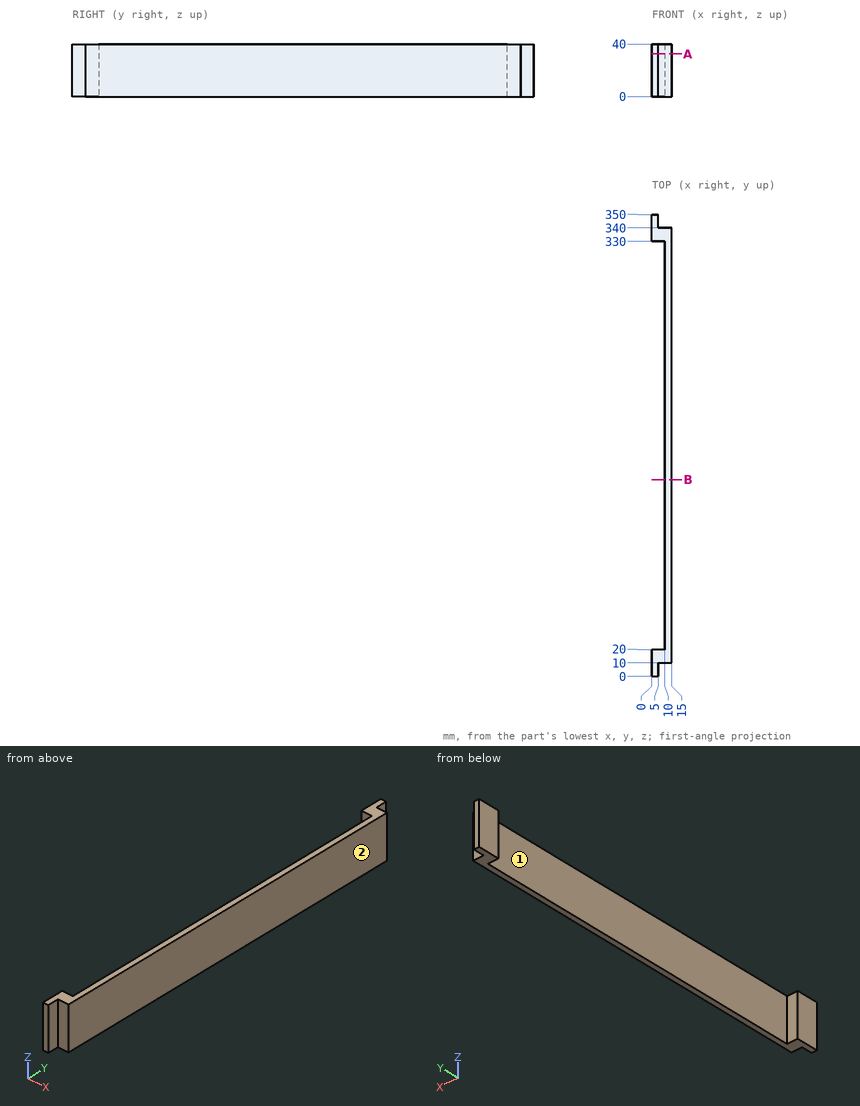
Input: dimensioned drawing with shaded views. Units: mm. Origin: part minimum x, y, z. Give positions to 0.01 mm unless a question says otherwise; leave off trailing zeros. Loops run counter-clockwise (first coordinate to the right, second up) from the corner with the lowest first, then second, coordinate; pieces in that order, holes last. Notation, with made-up numbers: M 57.25,31 L 98.25,31 A18 cw 98.25,58 Z; hole C 25.25,23.25 d6. An arc over 180 degrees is marked long. Put each result on its own line as item: value. Start each with the question number.
1) Cut plane B-B (y = 149). Output: boundary loops of the cut face in (x, z).
2) Ray query, line 1 along Y through (x, z) = (6.5, 32.5); line 2 along Y through (x, z) = (3.75, 24.5); line 3 along Y through (x, z) = (12.25, 2). Return the intervals inside material, ascending.
3) Cut plane A-A (z = 32.5). Output: boundary loops of the cut face in (x, y), then the cut area to 3 significant figures.
4) Pull-direction query (Y, two-part tool) for the marked faces 1 and 2; classes: pulls with the +Y half, pulls with the -Y half, needs draft (parallel to the pull), parting line crosses it, or undercut.
5) Contact query for flat-ended pins moving along their axis: pin 1 (5 mm diameter, centred on y = 117, z = 6.5, fed in from -X); pin 2 (5 mm diameter, centred on x = 9, z = 23, fed in from +Y); pin 3 (5 mm diameter, centred on x = 9.5, z = 18.5, fed in from -Y). Output: stop coordinate, or through.
Verdict:
1. outline: M 10,0 L 15,0 L 15,40 L 10,40 Z
2. line 1: 10 to 20, 330 to 340
2. line 2: 0 to 20, 330 to 350
2. line 3: 10 to 340
3. outline: M 0,0 L 5,0 L 5,10 L 15,10 L 15,340 L 5,340 L 5,350 L 0,350 L 0,330 L 10,330 L 10,20 L 0,20 Z
3. area: 1,950 mm2
4. face 1: undercut
4. face 2: needs draft
5. pin 1: x = 10
5. pin 2: y = 340
5. pin 3: y = 10
